Design review of the part built by this model. Coordinates are the model's own, in mm. Give positions to 0.01 mm unless a question says otherwise; leave off trailing zeros. Write each loop counter-clockwise with the first axis right and the second up, starting at its lowest first coordinate (ties: lowest second). Pieces come first, ordered by that corner, then holes.
```python
from build123d import *

# Parameters (mm, degrees)
F0_W     = 93.98
F0_H     = 88.9
F0_R     = 1.5875
F0_R_2   = 2.413
F1_DEPTH = 5.842


with BuildPart() as f1:
    # F0 (on Front) → F1 (new body)
    with BuildSketch(Plane.XZ):
        with Locations((46.99, -44.45)):
            Rectangle(F0_W, F0_H)
        with Locations((6.096, -82.55)):
            Circle(F0_R, mode=Mode.SUBTRACT)
        with Locations((6.096, -73.025)):
            Circle(F0_R_2, mode=Mode.SUBTRACT)
        with Locations((17.6276, -62.4078)):
            Circle(F0_R, mode=Mode.SUBTRACT)
        with Locations((25.2476, -62.4078)):
            Circle(F0_R_2, mode=Mode.SUBTRACT)
        with Locations((69.596, -82.55)):
            Circle(F0_R, mode=Mode.SUBTRACT)
        with Locations((69.596, -73.025)):
            Circle(F0_R_2, mode=Mode.SUBTRACT)
        with Locations((80.01, -62.4078)):
            Circle(F0_R_2, mode=Mode.SUBTRACT)
        with Locations((87.63, -62.4078)):
            Circle(F0_R, mode=Mode.SUBTRACT)
        with Locations((6.096, -21.971)):
            Circle(F0_R_2, mode=Mode.SUBTRACT)
        with Locations((6.096, -12.446)):
            Circle(F0_R, mode=Mode.SUBTRACT)
        with Locations((18.796, -21.971)):
            Circle(F0_R, mode=Mode.SUBTRACT)
        with Locations((18.796, -12.446)):
            Circle(F0_R_2, mode=Mode.SUBTRACT)
        with Locations((56.896, -21.971)):
            Circle(F0_R, mode=Mode.SUBTRACT)
        with Locations((56.896, -12.446)):
            Circle(F0_R_2, mode=Mode.SUBTRACT)
        with Locations((69.596, -21.971)):
            Circle(F0_R_2, mode=Mode.SUBTRACT)
        with Locations((69.596, -12.446)):
            Circle(F0_R, mode=Mode.SUBTRACT)
    extrude(amount=F1_DEPTH)


solid = f1.part
```
(1) Consider section B-B, the plane z = -82.55. Give the boundary of the cut face in (x, y), then the cut area to 3 significant figures.
Resolved:
outline: (0, -5.84) - (4.51, -5.84) - (4.51, 0) - (0, 0) - close; (7.68, -5.84) - (68.01, -5.84) - (68.01, 0) - (7.68, 0) - close; (71.18, -5.84) - (93.98, -5.84) - (93.98, 0) - (71.18, 0) - close
area: 512 mm2
(2) To check wall thickness, follow L1, parallel to Z at x = 20, y = -4.25; L2, parallel to X at y = -4.85, z = -63; L3, parallel to X at y = -3.25, z = -21.5. State the ranges of each line that lie inside material, in increasing order.
Resolved:
L1: z = -88.9 to -23.01, -20.94 to -14.54, -10.35 to 0
L2: x = 0 to 16.15, 19.1 to 22.91, 27.59 to 77.67, 82.35 to 86.16, 89.1 to 93.98
L3: x = 0 to 3.73, 8.46 to 17.28, 20.31 to 55.38, 58.41 to 67.23, 71.96 to 93.98
(3) Consider section C-C, the plane y = -3.3. Give the number of separate pieces and of enclosed holes in the cut face, then the cut area to 3 significant figures.
Resolved:
separate pieces: 1
enclosed holes: 16
area: 8,150 mm2
(4) Mouldability with a two-part tool opening along Z and no side actions: class faces 1 (the face through (71.825, -2.88, -22.895)), 2 (the face through (46, -3, 0)), 3 (the face through (46, -5.842, -44)), 4 (the face through (71.062, -2.88, -13.054)) as pulls with the +Z half, pulls with the -Z half, needs draft (parallel to the pull), parting line crosses it, or undercut.
Resolved:
face 1: undercut
face 2: pulls with the +Z half
face 3: needs draft
face 4: undercut
(5) Consider section A-A, the plane x = 87.63. Give the boundary of the cut face in (y, z), then the cut area to 3 significant figures.
Resolved:
outline: (-5.84, -88.9) - (0, -88.9) - (0, -64) - (-5.84, -64) - close; (-5.84, -60.82) - (0, -60.82) - (0, 0) - (-5.84, 0) - close
area: 501 mm2
